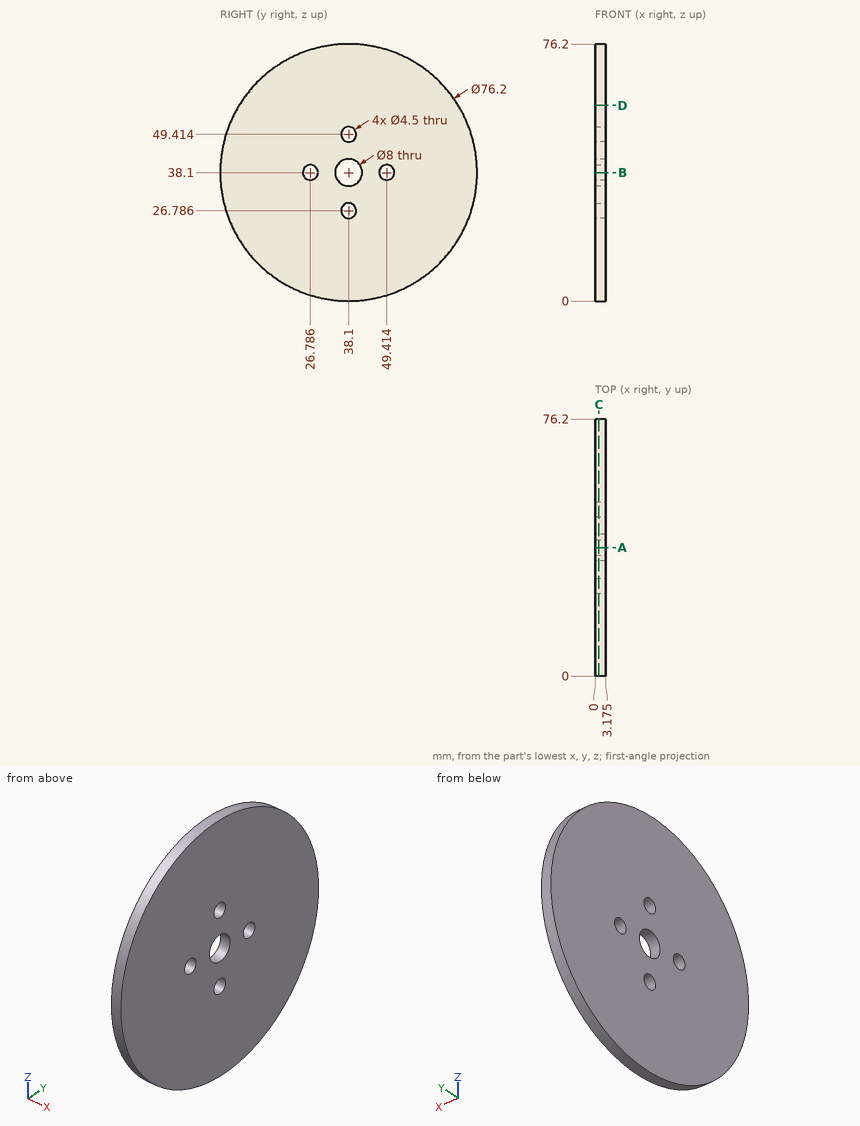
Source: three-view drawing plus pictorial views. Frame: mm from the lowest corner of the part. Round coordinates to 2 decimals unless told otherwise and drop trailing zeros. Loops run counter-clockwise (first coordinate to the right, second up) from the corner with the lowest first, then second, coordinate; pieces in that order, holes last. Notation, with made-up numbers: (84, 77.5) - (98, 77.5) arc R27 ccw to (98, 102.5) - close; hole circle Ø11 at (-2, -2.5). An arc over 180 degrees is marked (long way). Write item = value, one per line. Start each with the question number.
Item 1: Section query A-A on y = 38.1. Output: boundary loops of the cut face in (x, z) (1 decimal), plus the area to 3 significant figures.
Item 2: Material intervals for line 1 (Y direction, x = 1.4, z = 38.1); line 2 (Z direction, x = 0.9, y = 28) (1 decimal); line 3 (Z direction, x = 2.4, y = 49), sorted ascending.
Item 3: First-contact query: pin 1 Ø1 at (x, z) = (1, 13.5) entering from -Y; pin 2 Ø2.5 at (y, z) = (49.41, 38.1) entering from +X; pin 3 Ø1 at (x, y) = (2, 16) entering from +Z (1 decimal); pin 4 Ø1.5 at (x, z) = (3, 52) entering from -Y. Flat tips, straight axial feed; report the tip coordinate or a pass-through.
Item 4: Section query D-D on z = 58. Output: boundary loops of the cut face in (x, y) (1 decimal).
Item 5: Section query C-C on x = 1.1. Output: boundary loops of the cut face in (y, z), plus the area to 3 significant figures.
Results list:
q1.outline = (0, 0) - (3.2, 0) - (3.2, 24.5) - (0, 24.5) - close; (0, 29) - (3.2, 29) - (3.2, 34.1) - (0, 34.1) - close; (0, 42.1) - (3.2, 42.1) - (3.2, 47.2) - (0, 47.2) - close; (0, 51.7) - (3.2, 51.7) - (3.2, 76.2) - (0, 76.2) - close
q1.area = 188 mm²
q2.line_1 = 0 to 24.54, 29.04 to 34.1, 42.1 to 47.16, 51.66 to 76.2
q2.line_2 = 1.4 to 36.2, 40 to 74.8
q2.line_3 = 1.59 to 35.89, 40.31 to 74.61
q3.pin_1 = 8.59
q3.pin_2 = through
q3.pin_3 = 69.5
q3.pin_4 = 2.34
q4.outline = (0, 5.6) - (3.2, 5.6) - (3.2, 70.6) - (0, 70.6) - close
q5.outline = circle Ø76.2 at (38.1, 38.1); hole circle Ø4.5 at (26.79, 38.1); hole circle Ø8 at (38.1, 38.1); hole circle Ø4.5 at (38.1, 26.79); hole circle Ø4.5 at (38.1, 49.41); hole circle Ø4.5 at (49.41, 38.1)
q5.area = 4,450 mm²
